Can you work these out from the drawing? Everything is in mm from the part's minimum corner. A direction names the side the tool comes from. Give positions to 0.01 mm unless a question says otherwise; leave off trailing zeros. Order: outer loops, then holes, each group sorted by start corner. A loop starts at its lowest first (then second) coordinate and runs counter-clockwise, first axis right, second up. Notation, with made-up numbers: (-7.75, 43.25) -> (5.25, 43.25) arc R4 ccw to (5.25, 47.25) -> close; hole circle Ø1 at (49, -22). An arc over 180 degrees is marked (long way). Answer as CSV lines item,"result". Start each with the question number.
(1) I want a section at D-D (y = 7.5). Please give me the cut outline in (x, z), plus the area to 3 significant figures.
(2) I want a section at C-C (x = 6). Please give me the cut outline in (y, z), plus the area to 3 significant figures.
(3) I want a section at A-A (y = 20.5). Please give me the cut outline in (x, z), plus the area to 3 significant figures.
(4) On a 3-axis mill with a long thin cutter (end or side, diameter ignored), from which of +Z, -Z, +X, -X, +Y, -Y can I reach the whole of each face in a straight line? I mean the marked faces 1 and 2. Say none if no direction works.
(5) Will these pins go through, and if not, where does the flat tip stop? pin 1 Ø2.5 at (x, z) = (6, 8) entering from -Y; pin 2 Ø4 at (y, z) = (15, 2.5) entering from -X; pin 3 Ø2 at (y, z) = (23.5, 15.5) entering from -X; pin 4 Ø8 at (x, z) = (10.5, 7.5) entering from +Y.
(6) I want a section at B-B (z = 8). Please give me the cut outline in (x, y), plus the area to 3 significant figures.
(7) I need wall thicknesses on L1, parallel to X at y = 6, z = 8; L2, parallel to Z at x = 7, y = 21.5; L3, parallel to Y at x = 0.5, z = 11. Which ranges of each line are inside material? Lowest first, please.
(8) We'd pull the mould along Z, two halves only. Please class the marked faces 3, 4 and 5: released by +Z, released by -Z, zero draft, split by the parting line, or undercut.
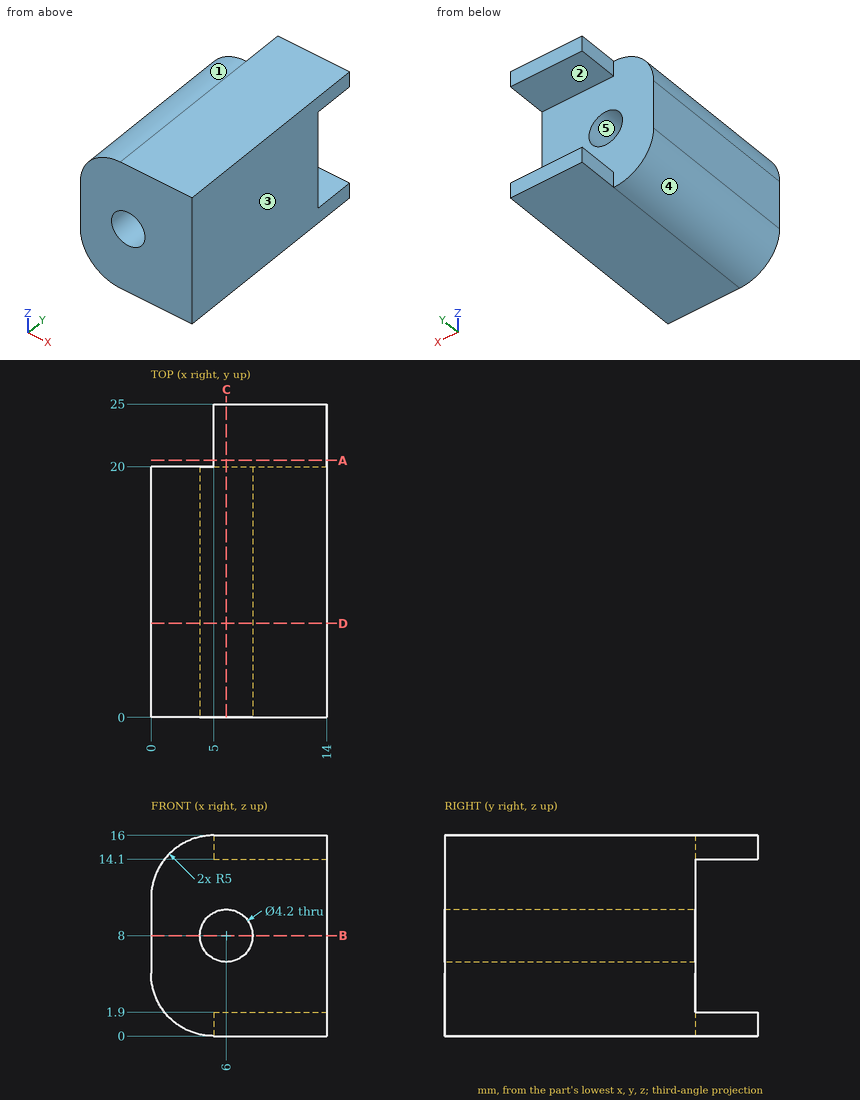
Final values:
1,outline,"(0, 5) arc R5 ccw to (5, 0) -> (14, 0) -> (14, 16) -> (5, 16) arc R5 ccw to (0, 11) -> close; hole circle Ø4.2 at (6, 8)"
1,area,"199 mm²"
2,outline,"(0, 0) -> (25, 0) -> (25, 1.9) -> (20, 1.9) -> (20, 5.9) -> (0, 5.9) -> close; (0, 10.1) -> (20, 10.1) -> (20, 14.1) -> (25, 14.1) -> (25, 16) -> (0, 16) -> close"
2,area,"255 mm²"
3,outline,"(5, 0) -> (14, 0) -> (14, 1.9) -> (5, 1.9) -> close; (5, 14.1) -> (14, 14.1) -> (14, 16) -> (5, 16) -> close"
3,area,"34.2 mm²"
4,face 1,"+Z, -X, +Y, -Y"
4,face 2,"+X, -X, +Y"
5,pin 1,"through"
5,pin 2,"x = 0.03"
5,pin 3,"x = 5"
5,pin 4,"y = 20"
6,outline,"(0, 0) -> (3.9, 0) -> (3.9, 20) -> (0, 20) -> close; (8.1, 0) -> (14, 0) -> (14, 20) -> (8.1, 20) -> close"
6,area,"196 mm²"
7,L1,"0 to 3.9, 8.1 to 14"
7,L2,"0 to 1.9, 14.1 to 16"
7,L3,"0 to 20"
8,face 3,"zero draft"
8,face 4,"released by -Z"
8,face 5,"undercut"
